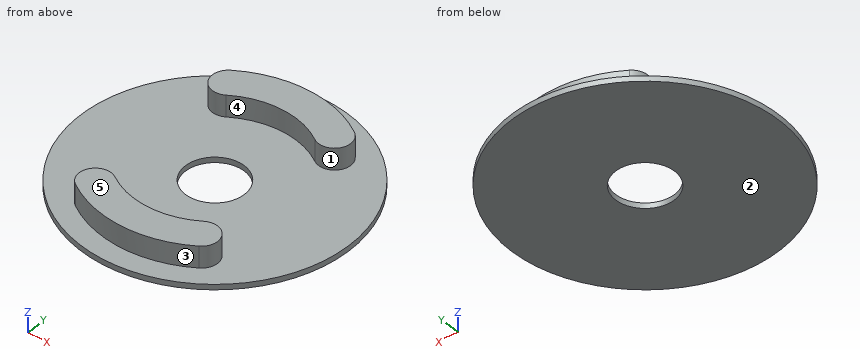
from build123d import *

# Parameters (mm, degrees)
SKETCH002_R   = 25
SKETCH002_R_2 = 5.5
PAD_DEPTH     = 1
PAD001_DEPTH  = 4


with BuildPart() as part:
    # Sketch002 → Pad (new body)
    with BuildSketch(Plane.XY):
        Circle(SKETCH002_R)
        Circle(SKETCH002_R_2, mode=Mode.SUBTRACT)
    extrude(amount=PAD_DEPTH)

    # Sketch001 → Pad001 (join)
    with BuildSketch(Plane.XY.offset(1)):
        with BuildLine():
            ThreePointArc((8.351648, 12.699999), (0, 15.2), (-8.351648, 12.699999))
            ThreePointArc((-11.648352, 17.713156), (-12.506579, 13.558226), (-8.351648, 12.699999))
            ThreePointArc((11.648352, 17.713156), (0, 21.2), (-11.648352, 17.713156))
            ThreePointArc((8.351648, 12.699999), (12.506579, 13.558226), (11.648352, 17.713156))
        make_face()
        with BuildLine():
            ThreePointArc((-8.351648, -12.699999), (0, -15.2), (8.351648, -12.699999))
            ThreePointArc((11.648352, -17.713156), (12.506579, -13.558226), (8.351648, -12.699999))
            ThreePointArc((-11.648352, -17.713156), (0, -21.2), (11.648352, -17.713156))
            ThreePointArc((-8.351648, -12.699999), (-12.506579, -13.558226), (-11.648352, -17.713156))
        make_face()
    extrude(amount=PAD001_DEPTH)


solid = part.part
Input: part model. Units: mm. Frame: model coordinates. Face numbers are marked on the shaded views. A direction names the side the tool comes from. Give positions to 0.01 mm unless a question says otherwise; leave off trailing zeros. Order: outer loops, then holes, each group sorted by start corner. A loop starts at its lowest first (then second) coordinate and runs counter-clockwise, first axis right, second up. Notation, with made-up numbers: M -12.5,-12.75 L 27.5,-12.75 A10 ccw 27.5,-6.75 Z; hole C 56.5,-31 d3. An arc over 180 degrees is marked long. Answer as a JSON object with one key per item and string values.
1. Cut plane A-A, the plane x = 0. Output: boundary loops of the cut face in (y, z).
Result sheet:
{"outline": "M -25,0 L -5.5,0 L -5.5,1 L -15.2,1 L -15.2,5 L -21.2,5 L -21.2,1 L -25,1 Z; M 5.5,0 L 25,0 L 25,1 L 21.2,1 L 21.2,5 L 15.2,5 L 15.2,1 L 5.5,1 Z"}
2. Cut plane D-D, the plane x = 10. Output: boundary loops of the cut face in (y, z).
Result sheet:
{"outline": "M -22.91,0 L 22.91,0 L 22.91,1 L 18.69,1 L 18.69,5 L 12.21,5 L 12.21,1 L -12.21,1 L -12.21,5 L -18.69,5 L -18.69,1 L -22.91,1 Z"}
3. First-contact query: P1, Ø1.5, axis at x = -18, y = -2, coming from the +Z side. Flat tip, straight axial feed; report the tip coordinate or a pass-through.
Result sheet:
{"P1": "z = 1"}
4. Pull-direction query (X, two-part tool) for the marked faces 3, 4 and 5; classes: +X half, -X half, draft (parallel to the pull), parting line (faces both ways), or undercut.
Result sheet:
{"face 3": "parting line", "face 4": "undercut", "face 5": "draft"}
5. Reachability of the marked faces 1 and 2 from +Z, -Z, +X, -X, +Y, -Y: full face, straight path, thin tool, end or side. Return the list, or none.
Result sheet:
{"face 1": "+Z", "face 2": "-Z, +X, -X, +Y, -Y"}
6. Cut plane B-B, the plane z = 1.9. Output: boundary loops of the cut face in (x, y).
Result sheet:
{"outline": "M -11.65,-17.71 A21.2 ccw 11.65,-17.71 A3 ccw 8.35,-12.7 A15.2 cw -8.35,-12.7 A3 ccw Z; M -11.65,17.71 A3 ccw -8.35,12.7 A15.2 cw 8.35,12.7 A3 ccw 11.65,17.71 A21.2 ccw Z"}
7. Ray query, line 1 (Z direction, x = 21.5, y = 5.5); line 2 (Y direction, x = 0, z = 0.45); line 3 (Y direction, x = -10, z = 4.45). Return the intervals inside material, ascending. Write a range as [from, to].
Result sheet:
{"line 1": "[0, 1]", "line 2": "[-25, -5.5], [5.5, 25]", "line 3": "[-18.69, -12.21], [12.21, 18.69]"}
8. Cut plane C-C, the plane y = 0. Output: boundary loops of the cut face in (x, z).
Result sheet:
{"outline": "M -25,0 L -5.5,0 L -5.5,1 L -25,1 Z; M 5.5,0 L 25,0 L 25,1 L 5.5,1 Z"}
